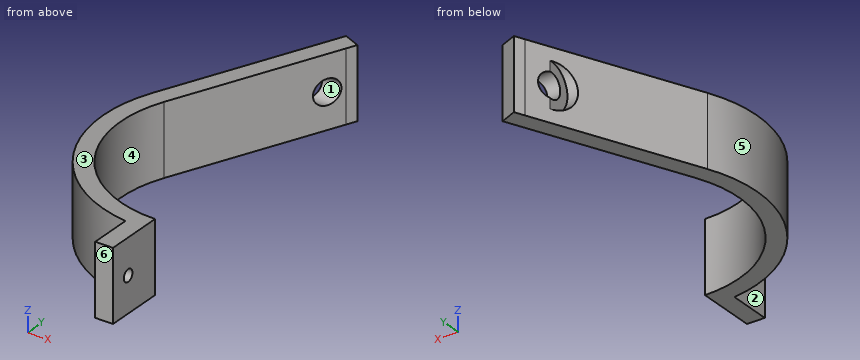
```python
from build123d import *

# Parameters (mm, degrees)
F1_DEPTH  = 20
F2_R      = 3.4925
F3_DEPTH  = 50
F5_R      = 6.35
F5_R_2    = 3.4925
F6_DEPTH  = 7
F7_W      = 56.608487
F7_H      = 135.039326
F8_DEPTH  = 25
F9_R      = 1.7
F10_DEPTH = 25
F12_DEPTH = 25
F14_DEPTH = 20


with BuildPart() as f1:
    # F0 (on Top) → F1 (new body)
    with BuildSketch(Plane.XY):
        with BuildLine():
            ThreePointArc((15.308536, 92.973734), (0, 103), (-15.308536, 92.973734))
            Line((-15.308536, 92.973734), (-34.833795, 48.185741))
            ThreePointArc((-34.833795, 48.185741), (-33.092371, 14.321269), (-5, -4.669616))
            Line((-5, -4.669616), (-5, -16.669616))
            Line((-5, -16.669616), (0, -16.669616))
            Line((0, -16.669616), (0, -5))
            ThreePointArc((0, -5), (31.78882, 12.180036), (34.833795, 48.185741))
            Line((34.833795, 48.185741), (15.308536, 92.973734))
        make_face()
        with BuildLine():
            ThreePointArc((-10.725142, 90.97561), (0, 98), (10.725142, 90.97561))
            Line((10.725142, 90.97561), (30.250401, 46.187617))
            ThreePointArc((30.250401, 46.187617), (0, 0), (-30.250401, 46.187617))
            Line((-30.250401, 46.187617), (-10.725142, 90.97561))
        make_face(mode=Mode.SUBTRACT)
    extrude(amount=F1_DEPTH)

    # F2 (on Right) → F3 (cut, symmetric)
    with BuildSketch(Plane.YZ):
        with Locations((86.3, 10)):
            Circle(F2_R)
    extrude(amount=F3_DEPTH, both=True, mode=Mode.SUBTRACT)

    # F5 (on offset) → F6 (cut)
    with BuildSketch(Plane.YZ.offset(-25)):
        with Locations((86.3, 10)):
            Circle(F5_R)
        with Locations((86.3, 10)):
            Circle(F5_R_2, mode=Mode.SUBTRACT)
    extrude(amount=F6_DEPTH, mode=Mode.SUBTRACT)

    # F7 (on face) → F8 (cut)
    with BuildSketch(Plane.XY.offset(20)):
        with Locations((28.304243, 38.84458)):
            Rectangle(F7_W, F7_H)
    extrude(amount=-F8_DEPTH, mode=Mode.SUBTRACT)

    # F9 (on face) → F10 (cut)
    with BuildSketch(Plane(origin=(-5, 0, 0), x_dir=(0, -1, 0), z_dir=(-1, 0, 0))):
        with Locations((10.669616, 10)):
            Circle(F9_R)
    extrude(amount=-F10_DEPTH, mode=Mode.SUBTRACT)

    # F11 (on face) → F12 (cut)
    with BuildSketch(Plane.XY.offset(20)):
        Polygon((-17.911747, 98.920211), (-15.308536, 92.973734), (-10.725142, 90.97561), (6.21896, 97.293422), (0, 104.071707), align=None)
    extrude(amount=-F12_DEPTH, mode=Mode.SUBTRACT)

    # F13 (on Top) → F14 (join)
    with BuildSketch(Plane.XY):
        Polygon((-14.109662, 95.72377), (-15.308536, 92.973734), (-10.725142, 90.97561), (-9.526268, 93.725646), align=None)
    extrude(amount=F14_DEPTH)


solid = f1.part
```
The listing builds one solid part. Answer for the finished solid, in the listing's coordinates (mm). Face numbers are marked on the shaded views. A direction names the side the tool comes from. Round coordinates to 2 decimals unless told otherwise and drop trailing zeros. Loops run counter-clockwise (first coordinate to the right, second up) from the corner with the lowest first, then second, coordinate; pieces in that order, holes last. Notation, with made-up numbers: (85, -38) - (103, -38) arc R9 ccw to (103, -28) - close; hole circle Ø3 at (-20, -15.75). An arc over 180 degrees is marked (long way). Use one line per item in the form item = value. Start each with the question number.
1. The part is cut by section B-B on y = 35. Determine the outline of the cut face in (x, z), then the cut area to 3 significant figures.
2. For a pull along Y with two mould halves and no side action, classify the marked faces 3, 4, 5 and 6 as pulls with the +Y half, pulls with the -Y half, needs draft (parallel to the pull), parting line crosses it, or undercut.
3. Consider line 1 (Z direction, x = -14.5, y = 86.3); line 2 (Y direction, x = -14.75, z = 10); line 3 (Y direction, x = -17, z = 2). Determine where each line is inside the solid, lowest interval first. Write a range as [from, to].
4. Given pin 1 Ø2 at (x, z) = (-34, 14.5) entering from -Y; pin 2 Ø9.5 at (y, z) = (-12, 6.5) entering from -X; pin 3 Ø4 at (y, z) = (65, 12.5) entering from +X, each flat-ended and moving along its own axis, determine where each tip first touches the part or whether it passes through.
5. A tool of negligible diameter and unlimited length cuts with its end or side. For the marked faces 1 and 2, from which of +Z, -Z, +X, -X, +Y, -Y can it reach the whole face along a straight path? Write none if from no direction.
6. The part is cut by section A-A on z = 10. Determine the outline of the cut face in (x, y), then the cut area to 3 significant figures.
7. The part is cut by section C-C on x = -8.5. Determine the outline of the cut face in (y, z).
Geometry check:
q1.outline = (-37.95, 0) - (-32.94, 0) - (-32.94, 20) - (-37.95, 20) - close
q1.area = 100 mm^2
q2.face_3 = needs draft
q2.face_4 = undercut
q2.face_5 = parting line crosses it
q2.face_6 = pulls with the -Y half
q3.line_1 = [0, 6.51], [13.49, 20]
q3.line_2 = [-2.02, 3.48], [81.74, 82.81], [89.79, 94.25]
q3.line_3 = [-0.99, 4.72], [76.58, 89.09]
q4.pin_1 = 14.16
q4.pin_2 = -5
q4.pin_3 = -21.18
q5.face_1 = +X, -X
q5.face_2 = +Z, -Z, -X, -Y
q6.outline = (-34.83, 48.19) arc R38 ccw to (-5, -4.67) - (-5, -8.97) - (0, -8.97) - (0, 0) arc R33 cw to (-30.25, 46.19) - (-14.29, 82.81) - (-18, 82.81) - (-18, 79.95) - (-20.99, 79.95) - close; (-16.7, 89.79) - (-11.24, 89.79) - (-9.53, 93.73) - (-14.11, 95.72) - close; (-5, -16.67) - (0, -16.67) - (0, -12.37) - (-5, -12.37) - close
q6.area = 608 mm^2
q7.outline = (-4.04, 0) - (1.11, 0) - (1.11, 20) - (-4.04, 20) - close
